Part model, mm, in its own coordinate system. A direction names the side the tool comes from. Coordinates: 2 decimals unless noted, no trailing zeros. Loops run counter-clockwise (first coordinate to the right, second up) from the corner with the lowest first, then second, coordinate; pieces in that order, holes last. Notation, with made-up numbers: (66, 33) -> (117, 33) arc R14 cw to (117, 57) -> close; hole circle Ø5 at (-39, 2.25). An arc over 180 degrees is marked (long way). One line per item, written item: value. Start each with the question number.
from build123d import *

# Parameters (mm, degrees)
BOSS_EXTRUDE1_DEPTH = 20.066
BOSS_EXTRUDE2_DEPTH = 2.54
SKETCH3_R           = 6.5405
BOSS_EXTRUDE3_DEPTH = 2.032
SKETCH4_R           = 2.921
BOSS_EXTRUDE4_DEPTH = 4.064


with BuildPart() as part:
    # Sketch1 → Boss-Extrude1 (new body)
    with BuildSketch(Plane.XY):
        Polygon((0, 0), (40.64, 0), (40.64, 28.575), (47.625, 28.575), (47.625, 30.988), (40.64, 30.988), (40.64, 36.83), (0, 36.83), (0, 30.988), (-6.985, 30.988), (-6.985, 28.575), (0, 28.575), align=None)
    extrude(amount=BOSS_EXTRUDE1_DEPTH)

    # Sketch2 → Boss-Extrude2 (add)
    with BuildSketch(Plane(origin=(0, 36.83, 0), x_dir=(1, 0, 0), z_dir=(0, 1, 0))):
        with BuildLine():
            Line((14.560242732, -1.0795), (33.655, -1.0795))
            Line((33.655, -1.0795), (33.655, -5.2705))
            ThreePointArc((33.655, -5.2705), (35.941, -10.033), (33.655, -14.7955))
            Line((33.655, -14.7955), (33.655, -18.9865))
            Line((33.655, -18.9865), (14.560242732, -18.9865))
            ThreePointArc((14.560242732, -18.9865), (0, -10.033), (14.560242732, -1.0795))
        make_face()
    extrude(amount=BOSS_EXTRUDE2_DEPTH)

    # Sketch3 → Boss-Extrude3 (add)
    with BuildSketch(Plane(origin=(0, 39.37, 0), x_dir=(1, 0, 0), z_dir=(0, 1, 0))):
        with Locations((10.033, -10.033)):
            Circle(SKETCH3_R)
    extrude(amount=BOSS_EXTRUDE3_DEPTH)

    # Sketch4 → Boss-Extrude4 (add)
    with BuildSketch(Plane(origin=(0, 41.402, 0), x_dir=(1, 0, 0), z_dir=(0, 1, 0))):
        with Locations((10.033, -10.033)):
            Circle(SKETCH4_R)
    extrude(amount=BOSS_EXTRUDE4_DEPTH)


solid = part.part
1) Probe line 1 (Y direction, x = 40, z = 8.25); line 2 (X direction, y = 21, z = 2.5); line 3 (Y direction, x = 30, z = 17.5). List the from-to ranges inside material, lowest first. Write a range as from..to.
2) Slice it at C-C (y = 4). Give the cut face in (x, z).
3) Slice it at B-B (z = 12.25). Give the cut face in (x, y) (3 decimals), then the cut area to 3 significant figures.
4) Pin check, flat tips, straight feed: pin 1 Ø0.8 at (y, z) = (37.5, 17) entering from +X (3 decimals); pin 2 Ø2 at (x, z) = (-4.5, 6.5) entering from -Y (3 decimals); pin 3 Ø5 at (x, z) = (2.5, 3.5) entering from +Y; pin 4 Ø2 at (x, y) = (24, 37.5) entering from -Z. Stop position of each tip, or through.
5) Slice it at D-D (x = 11). Give the cut face in (y, z), then the cut area to 3 significant figures.
6) Slice it at A-A (x = 25.5). Give the cut face in (y, z).
7) Tool access for faces 1 (the flat face through (11, 41.402, 13)), 2 (the flat face through (0, 14, 10)), 3 (the flat face through (0, 34, 10)): list every direction of +Z, -Z, +X, -X, +Y, -Y with a clear straight run to the whole face (end or side of a thin tool).
Check sheet entries:
1. line 1: y = 0..36.83
1. line 2: x = 0..40.64
1. line 3: y = 0..39.37
2. outline: (0, 0) -> (40.64, 0) -> (40.64, 20.07) -> (0, 20.07) -> close
3. outline: (-6.985, 28.575) -> (0, 28.575) -> (0, 0) -> (40.64, 0) -> (40.64, 28.575) -> (47.625, 28.575) -> (47.625, 30.988) -> (40.64, 30.988) -> (40.64, 36.83) -> (35.524, 36.83) -> (35.524, 39.37) -> (16.186, 39.37) -> (16.186, 41.402) -> (11.935, 41.402) -> (11.935, 45.466) -> (8.131, 45.466) -> (8.131, 41.402) -> (3.88, 41.402) -> (3.88, 39.37) -> (0.248, 39.37) -> (0.248, 36.83) -> (0, 36.83) -> (0, 30.988) -> (-6.985, 30.988) -> close
3. area: 1,660 mm^2
4. pin 1: stops at x = 33.655
4. pin 2: stops at y = 28.575
4. pin 3: stops at y = 39.37
4. pin 4: stops at z = 0
5. outline: (0, 0) -> (36.83, 0) -> (36.83, 0.05) -> (39.37, 0.05) -> (39.37, 3.56) -> (41.4, 3.56) -> (41.4, 7.28) -> (45.47, 7.28) -> (45.47, 12.79) -> (41.4, 12.79) -> (41.4, 16.5) -> (39.37, 16.5) -> (39.37, 20.02) -> (36.83, 20.02) -> (36.83, 20.07) -> (0, 20.07) -> close
5. area: 838 mm^2
6. outline: (0, 0) -> (36.83, 0) -> (36.83, 1.08) -> (39.37, 1.08) -> (39.37, 18.99) -> (36.83, 18.99) -> (36.83, 20.07) -> (0, 20.07) -> close
7. face 1: +Y
7. face 2: +Z, -Z, -X, -Y
7. face 3: +Z, -Z, -X, +Y
